Verification items for the finished model (mm, model axes). A direction names the side the tool comes from. Round coordinates to 2 decimals unless told otherwise and drop trailing zeros. Write each loop counter-clockwise with the first axis right and the second up, starting at its lowest first coordinate (ties: lowest second). Pieces come first, ordered by that corner, then holes. Notation, with made-up numbers: M -22,12.5 L -16,12.5 A31 cw -16,51.5 Z; hole C 25,-23.5 d11. An arc over 180 degrees is marked long. One line per item, written item: value. Start each with the question number.
Item 1: Thickness scan on probe 1 along X at (y, z) = (16.75, 182) (3 decimals); probe 2 along Y at (x, z) = (20.5, 66) (3 decimals); probe 3 along Y at (x, z) = (2, 138.5) (3 decimals). Record the ranges inside material, lowest first. Write a range as from..to.
Item 2: Section check C-C, the plane x = 7. Record the cut outline in (y, z) (3 decimals).
Item 3: Gauge pin test, flat ends, axial feed: pin 1 (4 mm diameter, centred on y = 15.875, z = 187.325, fed in from -X); pin 2 (4 mm diameter, centred on x = 22.5, z = 113, fed in from +Y) (3 decimals). Record the tip position at first contact, or that the pin passes through.
Item 4: Section check A-A, the plane y = 7.75. Record the cut outline in (x, z) (3 decimals), then the cut area to 3 significant figures.
Item 5: Draft check along Y on faces 3 (the face through (30.14, 17.09, 184.39)), 4 (the face through (15.735, 1.61, 165.097)), 5 (the face through (30, 28.575, 97)). Enter one of: +Y half, -Y half, draft (parallel to the pull), parting line (faces both ways), or undercut.
Item 6: Tool access check on faces 1 (the face through (31.75, 16, 97)), 2 (the face through (28.575, 17, 97)). Record the directions out of +Z, -Z, +X, -X, +Y, -Y that give a thin tool (end or side, any length) a straight path to the whole face; none if there is none.
Autodesk Inventor part; units mm, degrees
ref_plane "YZ Plane" through (0, 0, 0) normal (1, 0, 0) x (0, 1, 0)
ref_plane "XZ Plane" through (0, 0, 0) normal (0, 1, 0) x (-1, 0, 0)
ref_plane "XY Plane" through (0, 0, 0) normal (0, 0, 1) x (1, 0, 0)
sketch "Sketch1" plane through (0, 0, 0) normal (0, 0, 1) x (1, 0, 0)
  line L0 (3.175, 0) -> (28.575, 0)
  line L1 (31.75, 3.175) -> (31.75, 28.575)
  line L2 (0, 28.575) -> (0, 3.175)
  line L3 (4.7625, 3.175) -> (26.9875, 3.175)
  line L4 (28.575, 4.7625) -> (28.575, 28.575)
  line L5 (3.175, 28.575) -> (3.175, 4.7625)
  line L6 (0, 28.575) -> (3.175, 28.575)
  line L7 (28.575, 28.575) -> (31.75, 28.575)
  arc A0 (3.175, 4.7625) -> (4.7625, 3.175) centre (4.7625, 4.7625) ccw
  arc A1 (26.9875, 3.175) -> (28.575, 4.7625) centre (26.9875, 4.7625) ccw
  arc A2 (0, 3.175) -> (3.175, 0) centre (3.175, 3.175) ccw
  arc A3 (28.575, 0) -> (31.75, 3.175) centre (28.575, 3.175) ccw
  point P0 (0, 0)
  point P1 (0, 0)
  point P2 (31.75, 0)
  dimension "d0" = 31.75
  dimension "d1" = 28.575
  dimension "d2" = 1.5875
  dimension "d3" = 3.175
extrude "Extrusion1" add sketch "Sketch1" along normal blind 196.85
sketch "Sketch2" plane through (31.75, 3.175, 0) normal (1, 0, 0) x (0, 0, -1)
  line L0 (-196.85, 0) -> (-196.85, 25.4)
  line L1 (0, 0) -> (-196.85, 0)
  line L2 (-196.85, 12.7) -> (-187.325, 12.7)
  point P0 (0, -3.175)
  dimension "d6" = 9.525
sketch "Sketch3" plane through (3.175, 0, 0) normal (0, -1, 0) x (1, 0, 0)
  line L0 (0, 196.85) -> (25.4, 196.85)
  line L1 (0, 0) -> (0, 196.85)
  line L2 (12.7, 196.85) -> (12.7, 187.325)
  point P0 (-3.175, 0)
  dimension "d7" = 9.525
hole "Hole1" at (31.75, 15.875, 187.325) direction (-1, 0, 0) diameter 6.35 end through all
hole "Hole2" at (15.875, 0, 187.325) direction (0, 1, 0) diameter 6.35 end through all
pattern_linear "Rectangular Pattern1" count 8 spacing 25.4 along (0, 0, -1) of "Hole1", "Hole2"
properties part number "8 in bar"
Response values:
1. probe 1: x = 0..3.175, 28.575..31.75
1. probe 2: y = 0..3.175
1. probe 3: y = 0.225..13.389, 18.361..28.575
2. outline: M 0,0 L 3.175,0 L 3.175,196.85 L 0,196.85 Z
3. pin 1: passes through
3. pin 2: stops at y = 3.175
4. outline: M 0,0 L 3.175,0 L 3.175,196.85 L 0,196.85 Z; M 28.575,0 L 31.75,0 L 31.75,196.85 L 28.575,196.85 Z
4. area: 1,250 mm2
5. face 3: undercut
5. face 4: draft
5. face 5: +Y half
6. face 1: +Z, -Z, +X, +Y, -Y
6. face 2: +Z, -Z, +Y
